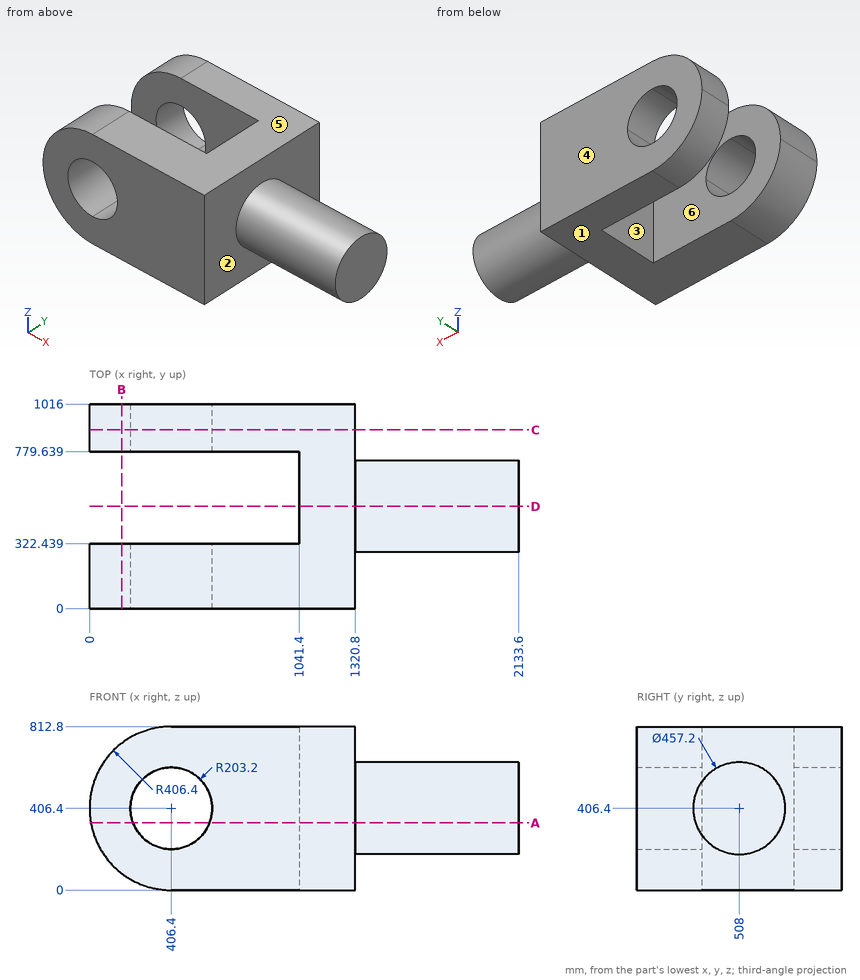
Input: dimensioned drawing with shaded views. Units: mm. Origin: part minimum x, y, z. A direction names the side the tool comes from. Round coordinates to 2 decimals unless told otherwise and drop trailing zeros. Loops run counter-clockwise (first coordinate to the right, second up) from the corner with the lowest first, then second, coordinate; pieces in that order, holes last. Notation, with made-up numbers: M -21.5,33.25 L 30.5,33.25 A20 ccw 30.5,42.25 Z; hole C -30.75,64 d9. An arc over 180 degrees is marked long. Answer in a Markdown table with one row per item. Add a question column.
1. Mould query, pull axis Y, two halves, no side actions, for the marked faces 4, 5 and 6. Classes: released by +Y, released by -Y, zero draft, split by the parting line, or undercut.
2. Ray query, probe 1 along Y at (x, z) = (998, 106); probe 2 along X at (y, z) = (531, 652.5); probe 3 along X at (y, z) = (537, 206.5). Return the intervals inside material, ascending.
3. Section D-D (y = 508). Output: boundary loops of the cut face in (x, z), and give its area (3 significant figures).
4. Set-up query: the marked faces 1, 2 and 3. Return all of +Z, -Z, +X, -X, +Y, -Y with unobstructed straight access to the full face (end or side cutting, diameter ignored); none if empty.
5. Section C-C (y = 887.5). Output: boundary loops of the cut face in (x, z), and give its area (3 significant figures).
6. Section A-A (z = 334). Output: boundary loops of the cut face in (x, y) (1 decimal), and give its area (3 significant figures).
7. Section B-B (x = 159). Output: boundary loops of the cut face in (y, z).
8. Contact query for flat-ended pins moving along their axis: pin 1 (2 mm diameter, centred on y = 274.5, z = 141, fed in from +X); pin 2 (4 mm diameter, centred on y = 107, z = 451, fed in from -X); pin 3 (2 mm diameter, centred on y = 238, z = 213.5, fed in from -X). Output: stop coordinate, or through.
Values follow:
| question | item | result |
|---|---|---|
| 1 | face 4 | released by +Y |
| 1 | face 5 | zero draft |
| 1 | face 6 | undercut |
| 2 | probe 1 | 0 to 322.44, 779.64 to 1016 |
| 2 | probe 2 | 1041.4 to 1320.8 |
| 2 | probe 3 | 1041.4 to 2133.6 |
| 3 | outline | M 1041.4,0 L 1320.8,0 L 1320.8,177.8 L 2133.6,177.8 L 2133.6,635 L 1320.8,635 L 1320.8,812.8 L 1041.4,812.8 Z |
| 3 | area | 599,000 mm^2 |
| 4 | face 1 | -Z, +X, -X, +Y, -Y |
| 4 | face 2 | +X |
| 4 | face 3 | +Z, -Z, -X |
| 5 | outline | M 406.4,0 L 1320.8,0 L 1320.8,812.8 L 406.4,812.8 A406.4 ccw Z; hole C 406.4,406.4 d406.4 |
| 5 | area | 873,000 mm^2 |
| 6 | outline | M 6.5,0 L 216.5,0 L 216.5,322.4 L 6.5,322.4 Z; M 6.5,779.6 L 216.5,779.6 L 216.5,1016 L 6.5,1016 Z; M 596.3,0 L 1320.8,0 L 1320.8,291.2 L 2133.6,291.2 L 2133.6,724.8 L 1320.8,724.8 L 1320.8,1016 L 596.3,1016 L 596.3,779.6 L 1041.4,779.6 L 1041.4,322.4 L 596.3,322.4 Z |
| 6 | area | 1,000,000 mm^2 |
| 7 | outline | M 0,83.98 L 322.44,83.98 L 322.44,728.82 L 0,728.82 Z; M 779.64,83.98 L 1016,83.98 L 1016,728.82 L 779.64,728.82 Z |
| 8 | pin 1 | x = 1320.8 |
| 8 | pin 2 | x = 2.24 |
| 8 | pin 3 | x = 48.16 |
